Verification items for this drawing (mm, ordinates from the low corner). A direction names the side the tool comes from. Round coordinates to 2 decimals unless told otherwise and drop trailing zeros. Order: outer loops, then holes, each group sorted by start corner. A loop starts at its lowest first (then second) coordinate and runs counter-clockwise, first axis right, second up. Notation, with made-up numbers: (-34.75, -33) -> (-2.75, -33) arc R19 ccw to (-2.75, -6) -> close; hole circle Ø2 at (44, 80). An arc over 180 degrees is marked (long way). Answer in a Markdown table with one row per item. Add a question column.
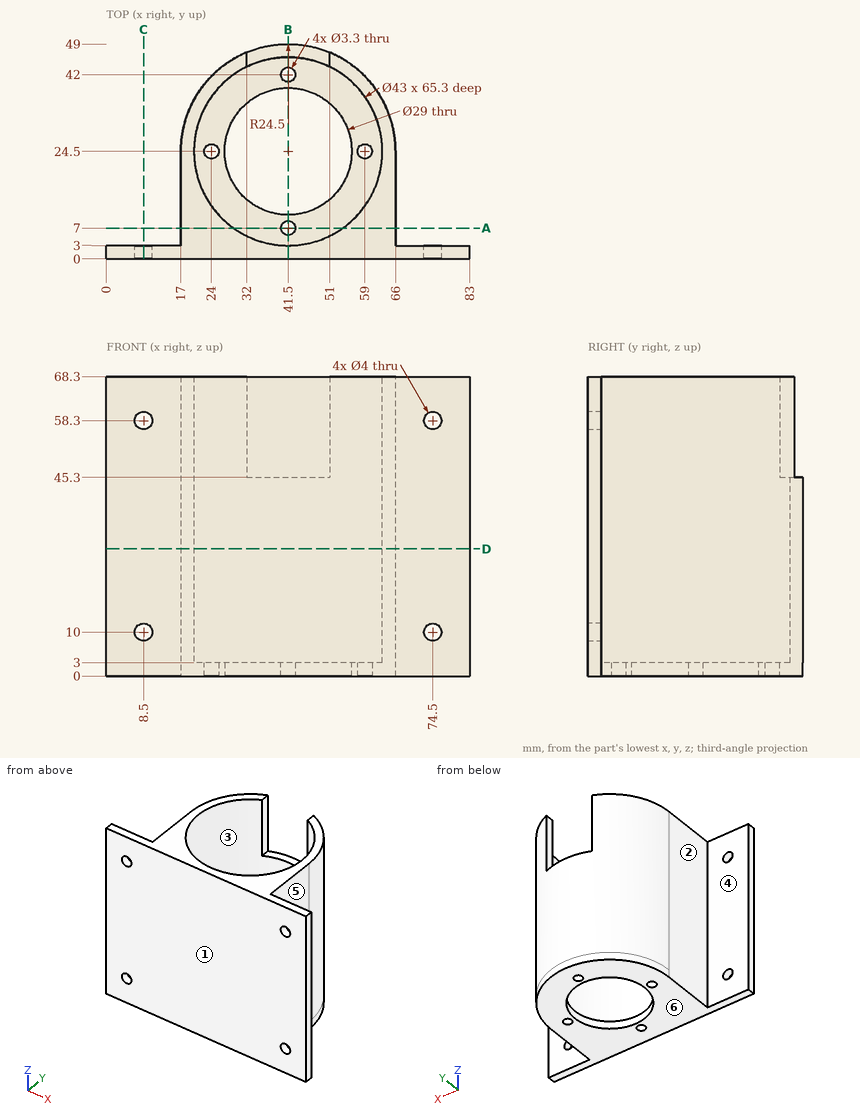
1) Tool access check on the marked faces 4, 5 and 6. Record the directions out of +Z, -Z, +X, -X, +Y, -Y that give a thin tool (end or side, any length) a straight path to the whole face; none if there is none.
2) Cross-section at B-B, the plane x = 41.5. Record the boundary of the cut face in (y, z), and give its area (3 significant figures).
3) Cross-section at A-A, the plane y = 7. Record the boundary of the cut face in (x, z).
4) Draft check along Y on the marked faces 1, 2 and 3. Enter one of: +Y half, -Y half, draft (parallel to the pull), parting line (faces both ways), or undercut.
5) Cross-section at C-C, the plane x = 8.5. Record the boundary of the cut face in (y, z).
6) Thickness scan on L1, parallel to X at y = 1.1, z = 10; L2, parallel to Y at x = 41.5, z = 1.4; L3, parallel to Z at x = 74, y = 1. Record the ranges inside material, lowest first. Write a range as [from, to].
7) Cross-section at D-D, the plane z = 29. Record the boundary of the cut face in (x, y), and give its area (3 significant figures).
8) Depth check by flat-ended pin: P1, Ø8, axis at x = 70.5, z = 60.5, coming from the -Y side; P2, Ø21.5, axis at x = 40.5, y = 19, coming from the +Z side; P3, Ø8.5, axis at x = 8.5, z = 43, coming from the +Y side; P4, Ø11, axis at y = 14, z = 24, coming from the -X side. Enter the tip coordinate at first touch or a pass-through.
Results below:
| question | item | result |
|---|---|---|
| 1 | face 4 | +Z, -Z, -X, +Y |
| 1 | face 5 | +Z, -Z, +X, +Y |
| 1 | face 6 | -Z, +X, -X, +Y, -Y |
| 2 | outline | (0, 0) -> (5.35, 0) -> (5.35, 3) -> (3, 3) -> (3, 68.3) -> (0, 68.3) -> close; (8.65, 0) -> (10, 0) -> (10, 3) -> (8.65, 3) -> close; (39, 0) -> (40.35, 0) -> (40.35, 3) -> (39, 3) -> close; (43.65, 0) -> (49, 0) -> (49, 45.3) -> (46, 45.3) -> (46, 3) -> (43.65, 3) -> close |
| 2 | area | 363 mm² |
| 3 | outline | (17, 0) -> (39.85, 0) -> (39.85, 3) -> (29.01, 3) -> (29.01, 68.3) -> (17, 68.3) -> close; (43.15, 0) -> (66, 0) -> (66, 68.3) -> (53.99, 68.3) -> (53.99, 3) -> (43.15, 3) -> close |
| 4 | face 1 | -Y half |
| 4 | face 2 | draft |
| 4 | face 3 | undercut |
| 5 | outline | (0, 0) -> (3, 0) -> (3, 8) -> (0, 8) -> close; (0, 12) -> (3, 12) -> (3, 56.3) -> (0, 56.3) -> close; (0, 60.3) -> (3, 60.3) -> (3, 68.3) -> (0, 68.3) -> close |
| 6 | L1 | [0, 6.5], [10.5, 72.5], [76.5, 83] |
| 6 | L2 | [0, 5.35], [8.65, 10], [39, 40.35], [43.65, 49] |
| 6 | L3 | [0, 8.06], [11.94, 56.36], [60.24, 68.3] |
| 7 | outline | (0, 0) -> (83, 0) -> (83, 3) -> (66, 3) -> (66, 24.5) arc R24.5 ccw to (17, 24.5) -> (17, 3) -> (0, 3) -> close; hole circle Ø43 at (41.5, 24.5) |
| 7 | area | 793 mm² |
| 8 | P1 | y = 0 |
| 8 | P2 | z = 3 |
| 8 | P3 | y = 3 |
| 8 | P4 | x = 17 |
